```python
from build123d import *

# Parameters (mm, degrees)
EXTRUDE_2_DEPTH     = 15
SKETCH_4_W          = 26
SKETCH_4_H          = 77
CUT_EXTRUDE_3_DEPTH = 10
CUT_EXTRUDE_5_DEPTH = 10
SKETCH_6_W          = 12
SKETCH_6_H          = 12
CUT_EXTRUDE_6_DEPTH = 4
SKETCH_7_W          = 2
SKETCH_7_H          = 2
EXTRUDE_5_DEPTH     = 3
SKETCH_8_W          = 2
SKETCH_8_H          = 1
EXTRUDE_6_DEPTH     = 7
SKETCH_9_R          = 1.75
CUT_EXTRUDE_7_DEPTH = 16


with BuildPart() as part:
    # ｽｹｯﾁ1 → ﾎﾞｽ - 押し出し2 (new body)
    with BuildSketch(Plane(origin=(0, 0, 0), x_dir=(0, 0, -1), z_dir=(1, 0, 0))):
        Polygon((25, 44.5), (25, -14.5), (45, -14.5), (45, -44.5), (25, -44.5), (-25, -44.5), (-25, 44.5), align=None)
    extrude(amount=EXTRUDE_2_DEPTH)

    # ｽｹｯﾁ4 → ｶｯﾄ - 押し出し3 (cut)
    with BuildSketch(Plane(origin=(15, 0, 0), x_dir=(0, 0, -1), z_dir=(1, 0, 0))):
        with Locations((0, 6)):
            Rectangle(SKETCH_4_W, SKETCH_4_H)
    extrude(amount=-CUT_EXTRUDE_3_DEPTH, mode=Mode.SUBTRACT)

    # ｽｹｯﾁ5 → ｶｯﾄ - 押し出し5 (cut)
    with BuildSketch(Plane(origin=(15, 0, 0), x_dir=(0, 0, -1), z_dir=(1, 0, 0))):
        with BuildLine():
            Line((13, -32.5), (13, -9.5))
            ThreePointArc((13, -9.5), (18.857864376, -23.642135624), (33, -29.5))
            Line((33, -29.5), (33, -32.5))
            Line((33, -32.5), (13, -32.5))
        make_face()
    extrude(amount=-CUT_EXTRUDE_5_DEPTH, mode=Mode.SUBTRACT)

    # ｽｹｯﾁ6 → ｶｯﾄ - 押し出し6 (cut)
    with BuildSketch(Plane(origin=(15, 0, 0), x_dir=(0, 0, -1), z_dir=(1, 0, 0))):
        with Locations((-19, 38.5)):
            Rectangle(SKETCH_6_W, SKETCH_6_H)
        with Locations((19, 38.5)):
            Rectangle(SKETCH_6_W, SKETCH_6_H)
    extrude(amount=-CUT_EXTRUDE_6_DEPTH, mode=Mode.SUBTRACT)

    # ｽｹｯﾁ7 → ﾎﾞｽ - 押し出し5 (add)
    with BuildSketch(Plane(origin=(5, 0, 0), x_dir=(0, 0, -1), z_dir=(1, 0, 0))):
        with Locations((-12, -31.5)):
            Rectangle(SKETCH_7_W, SKETCH_7_H)
        with Locations((32, -31.5)):
            Rectangle(SKETCH_7_W, SKETCH_7_H)
    extrude(amount=EXTRUDE_5_DEPTH)

    # ｽｹｯﾁ8 → ﾎﾞｽ - 押し出し6 (add)
    with BuildSketch(Plane(origin=(8, 0, 0), x_dir=(0, 0, -1), z_dir=(1, 0, 0))):
        with Locations((-12, -32)):
            Rectangle(SKETCH_8_W, SKETCH_8_H)
        with Locations((32, -32)):
            Rectangle(SKETCH_8_W, SKETCH_8_H)
    extrude(amount=EXTRUDE_6_DEPTH)

    # ｽｹｯﾁ9 → ｶｯﾄ - 押し出し7 (cut, through all)
    with BuildSketch(Plane(origin=(15, 0, 0), x_dir=(0, 0, -1), z_dir=(1, 0, 0))):
        with Locations((-19, 21.5)):
            Circle(SKETCH_9_R)
        with Locations((-19, -8.5)):
            Circle(SKETCH_9_R)
        with Locations((-19, -38.5)):
            Circle(SKETCH_9_R)
        with Locations((10, -38.5)):
            Circle(SKETCH_9_R)
        with Locations((39, -38.5)):
            Circle(SKETCH_9_R)
        with Locations((19, -8.5)):
            Circle(SKETCH_9_R)
        with Locations((19, 21.5)):
            Circle(SKETCH_9_R)
    extrude(amount=-CUT_EXTRUDE_7_DEPTH, mode=Mode.SUBTRACT)


solid = part.part
```
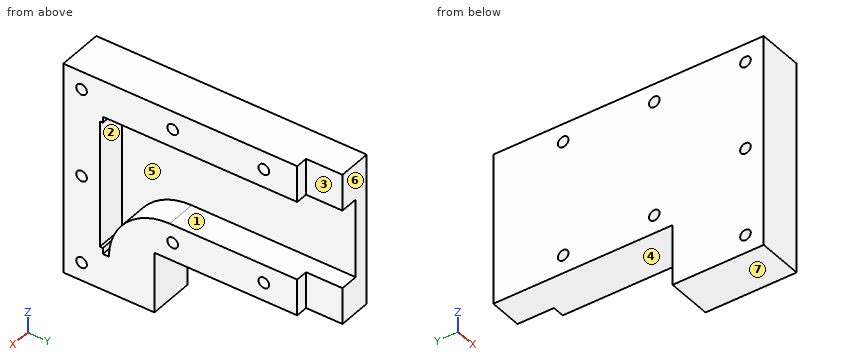
Geometry check sheet. Reference: the model listing, model coordinates, mm. Face numbers are marked on the shaded views. A direction names the side the tool comes from. Coordinates: 2 decimals unless noted, no trailing zeros. Loops run counter-clockwise (first coordinate to the right, second up) from the corner with the lowest first, then second, coordinate; pieces in that order, holes last. Notation, with made-up numbers: (81.25, -6.5) - (133.25, -6.5) arc R18 cw to (133.25, 11.5) - close; hole circle Ø4 at (85, 62). An arc over 180 degrees is marked (long way). One line per item, written item: value. Start each with the question number.
(1) Cross-section at A-A on y = -8.5. Enter the section's corners in (x, z).
(2) Tool access check on the marked faces 1, 2, 3 and 4. Record the directions out of +Z, -Z, +X, -X, +Y, -Y that give a thin tool (end or side, any length) a straight path to the whole face; none if there is none.
(3) Cross-section at C-C on z = 19. Enter the section's corners in (x, y), plus the area to 3 significant figures.
(4) Cross-section at B-B on x = 13. Enter the section's corners in (y, z).
(5) Material ranges on line 1 (Y direction, x = 8.75, z = 19); line 2 (Z direction, x = 3.5, y = -38); line 3 (Y direction, x = 10.75, z = -19), recorded low to high. Write a range as [from, to].
(6) Mould release check, pull along Z, two halves, no side actions. Record for the marked faces 5, 6 and 7: released by +Z, released by -Z, zero draft, split by the parting line, or undercut.
(7) Depth check by flat-ended pin: P1, Ø3, axis at x = 13.5, z = 21, coming from the +Y side; P2, Ø2, axis at y = -38.5, z = -39, coming from the -X side; P3, Ø1, axis at x = 12.5, z = -32.5, coming from the +Y side; P4, Ø5, axis at x = 12, y = 15, coming from the -Z side. Enter the tip coordinate at first touch or a pass-through.
(8) Cross-section at D-D on y = -38.5. Enter the section's corners in (x, z), plus the area to 4 significant figures.
Results below:
1. outline: (0, -25) - (15, -25) - (15, -20.75) - (0, -20.75) - close; (0, -17.25) - (15, -17.25) - (15, -13) - (5, -13) - (5, 13) - (15, 13) - (15, 17.25) - (0, 17.25) - close; (0, 20.75) - (15, 20.75) - (15, 25) - (0, 25) - close
2. face 1: +X, +Y
2. face 2: +X
2. face 3: +Z, -Z, +X, +Y
2. face 4: -Z, +X, -X, +Y
3. outline: (0, -44.5) - (15, -44.5) - (15, -40.25) - (0, -40.25) - close; (0, -36.75) - (15, -36.75) - (15, -10.25) - (0, -10.25) - close; (0, -6.75) - (15, -6.75) - (15, 19.75) - (0, 19.75) - close; (0, 23.25) - (15, 23.25) - (15, 32.5) - (11, 32.5) - (11, 44.5) - (0, 44.5) - close
3. area: 1,130 mm2
4. outline: (-44.5, -45) - (-14.5, -45) - (-14.5, -25) - (32.5, -25) - (32.5, -13) - (-9.5, -13) arc R20 ccw to (-29.5, -33) - (-31.5, -33) - (-31.5, -31) - (-32.5, -31) - (-32.5, 11) - (-31.5, 11) - (-31.5, 13) - (32.5, 13) - (32.5, 25) - (-44.5, 25) - close; hole circle Ø3.5 at (-38.5, -39); hole circle Ø3.5 at (-38.5, -10); hole circle Ø3.5 at (-38.5, 19); hole circle Ø3.5 at (-8.5, -19); hole circle Ø3.5 at (-8.5, 19); hole circle Ø3.5 at (21.5, -19); hole circle Ø3.5 at (21.5, 19)
5. line 1: y = [-44.5, -40.25], [-36.75, -10.25], [-6.75, 19.75], [23.25, 44.5]
5. line 2: z = [-45, -40.68], [-37.32, -11.68], [-8.32, 17.32], [20.68, 25]
5. line 3: y = [-44.5, -32.5], [-23.78, -10.25], [-6.75, 19.75], [23.25, 44.5]
6. face 5: undercut
6. face 6: zero draft
6. face 7: released by -Z
7. P1: stops at y = 32.5
7. P2: passes through
7. P3: stops at y = -14.5
7. P4: stops at z = -25
8. outline: (0, -45) - (15, -45) - (15, -40.75) - (0, -40.75) - close; (0, -37.25) - (15, -37.25) - (15, -11.75) - (0, -11.75) - close; (0, -8.25) - (15, -8.25) - (15, 17.25) - (0, 17.25) - close; (0, 20.75) - (15, 20.75) - (15, 25) - (0, 25) - close
8. area: 892.5 mm2
